from build123d import *

# Parameters (mm, degrees)
CROQUIS1_W               = 30
CROQUIS1_H               = 30
CROQUIS1_W_2             = 26
CROQUIS1_H_2             = 26
SALIENTE_EXTRUIR3_DEPTH  = 230
CROQUIS2_W               = 62.135011277
CROQUIS2_H               = 81.929382736
CORTAR_EXTRUIR3_DEPTH    = 28
CROQUIS3_R               = 2
CORTAR_EXTRUIR9_DEPTH    = 15
CROQUIS4_R               = 2
CORTAR_EXTRUIR10_DEPTH   = 15
CROQUIS5_W               = 30
CROQUIS5_H               = 30
CROQUIS5_W_2             = 26
CROQUIS5_H_2             = 26
SALIENTE_EXTRUIR6_DEPTH  = 12
CROQUIS7_W               = 18.119956634
CROQUIS7_H               = 38.019551867
SALIENTE_EXTRUIR7_DEPTH  = 2
CROQUIS8_W               = 19.256572939
CROQUIS8_H               = 35.130037486
SALIENTE_EXTRUIR8_DEPTH  = 2
CROQUIS9_R               = 2
CORTAR_EXTRUIR11_DEPTH   = 2
CROQUIS10_R              = 2
CORTAR_EXTRUIR12_DEPTH   = 2
CROQUIS11_W              = 68.798737931
CROQUIS11_H              = 42.92716572
CORTAR_EXTRUIR14_DEPTH   = 2
CROQUIS12_R              = 2
SALIENTE_EXTRUIR9_DEPTH  = 2
CROQUIS13_R              = 2
SALIENTE_EXTRUIR10_DEPTH = 2
CROQUIS14_R              = 1.5
CORTAR_EXTRUIR18_DEPTH   = 20
CROQUIS16_W              = 26
CROQUIS16_H              = 26
CROQUIS16_W_2            = 24
CROQUIS16_H_2            = 24
SALIENTE_EXTRUIR11_DEPTH = 212
CROQUIS17_R              = 1.5
CORTAR_EXTRUIR20_DEPTH   = 6
CROQUIS18_R              = 2.5
CORTAR_EXTRUIR21_DEPTH   = 2.25
CROQUIS19_W              = 30
CROQUIS19_H              = 30
CROQUIS19_W_2            = 24
CROQUIS19_H_2            = 24
SALIENTE_EXTRUIR12_DEPTH = 30
CROQUIS20_R              = 2
SALIENTE_EXTRUIR13_DEPTH = 2
CROQUIS21_R              = 2
SALIENTE_EXTRUIR14_DEPTH = 2
CROQUIS22_R              = 2
CORTAR_EXTRUIR22_DEPTH   = 52
CROQUIS23_R              = 2
CORTAR_EXTRUIR23_DEPTH   = 52
CROQUIS24_W              = 34.498036884
CROQUIS24_H              = 39.991384426
CORTAR_EXTRUIR24_DEPTH   = 5


with BuildPart() as part:
    # Croquis1 → Saliente-Extruir3 (new body)
    with BuildSketch(Plane(origin=(0, 0, 0), x_dir=(1, 0, 0), z_dir=(0, 1, 0))):
        Rectangle(CROQUIS1_W, CROQUIS1_H)
        Rectangle(CROQUIS1_W_2, CROQUIS1_H_2, mode=Mode.SUBTRACT)
    extrude(amount=SALIENTE_EXTRUIR3_DEPTH)

    # Croquis2 → Cortar-Extruir3 (cut)
    with BuildSketch(Plane(origin=(0, 230, 0), x_dir=(1, 0, 0), z_dir=(0, 1, 0))):
        with Locations((9.148629236, 2.703749702)):
            Rectangle(CROQUIS2_W, CROQUIS2_H)
    extrude(amount=-CORTAR_EXTRUIR3_DEPTH, mode=Mode.SUBTRACT)

    # Croquis3 → Cortar-Extruir9 (cut)
    with BuildSketch(Plane.XY.offset(15)):
        with Locations((3, 169)):
            Circle(CROQUIS3_R)
        with Locations((-3, 191)):
            Circle(CROQUIS3_R)
        with Locations((-3, 33)):
            Circle(CROQUIS3_R)
        with Locations((3, 11)):
            Circle(CROQUIS3_R)
    extrude(amount=-CORTAR_EXTRUIR9_DEPTH, mode=Mode.SUBTRACT)

    # Croquis4 → Cortar-Extruir10 (cut)
    with BuildSketch(Plane(origin=(0, 0, -15), x_dir=(-1, 0, 0), z_dir=(0, 0, -1))):
        with Locations((-3, 191)):
            Circle(CROQUIS4_R)
        with Locations((3, 169)):
            Circle(CROQUIS4_R)
        with Locations((3, 11)):
            Circle(CROQUIS4_R)
        with Locations((-3, 33)):
            Circle(CROQUIS4_R)
    extrude(amount=-CORTAR_EXTRUIR10_DEPTH, mode=Mode.SUBTRACT)

    # Croquis5 → Saliente-Extruir6 (add)
    with BuildSketch(Plane(origin=(0, 202, 0), x_dir=(1, 0, 0), z_dir=(0, 1, 0))):
        Rectangle(CROQUIS5_W, CROQUIS5_H)
        Rectangle(CROQUIS5_W_2, CROQUIS5_H_2, mode=Mode.SUBTRACT)
    extrude(amount=SALIENTE_EXTRUIR6_DEPTH)

    # Croquis7 → Saliente-Extruir7 (add)
    with BuildSketch(Plane.XY.offset(15)):
        with Locations((-0.954536797, 182.456683749)):
            Rectangle(CROQUIS7_W, CROQUIS7_H)
    extrude(amount=-SALIENTE_EXTRUIR7_DEPTH)

    # Croquis8 → Saliente-Extruir8 (add)
    with BuildSketch(Plane(origin=(0, 0, -15), x_dir=(-1, 0, 0), z_dir=(0, 0, -1))):
        with Locations((1.596533726, 178.910609938)):
            Rectangle(CROQUIS8_W, CROQUIS8_H)
    extrude(amount=-SALIENTE_EXTRUIR8_DEPTH)

    # Croquis9 → Cortar-Extruir11 (cut)
    with BuildSketch(Plane.XY.offset(15)):
        with Locations((-3, 203)):
            Circle(CROQUIS9_R)
        with Locations((3, 181)):
            Circle(CROQUIS9_R)
    extrude(amount=-CORTAR_EXTRUIR11_DEPTH, mode=Mode.SUBTRACT)

    # Croquis10 → Cortar-Extruir12 (cut)
    with BuildSketch(Plane(origin=(0, 0, -15), x_dir=(-1, 0, 0), z_dir=(0, 0, -1))):
        with Locations((-3, 203)):
            Circle(CROQUIS10_R)
        with Locations((3, 181)):
            Circle(CROQUIS10_R)
    extrude(amount=-CORTAR_EXTRUIR12_DEPTH, mode=Mode.SUBTRACT)

    # Croquis11 → Cortar-Extruir14 (cut)
    with BuildSketch(Plane(origin=(0, 214, 0), x_dir=(1, 0, 0), z_dir=(0, 1, 0))):
        with Locations((-6.144488578, -0.254830212)):
            Rectangle(CROQUIS11_W, CROQUIS11_H)
    extrude(amount=-CORTAR_EXTRUIR14_DEPTH, mode=Mode.SUBTRACT)

    # Croquis12 → Saliente-Extruir9 (add)
    with BuildSketch(Plane(origin=(0, 0, -15), x_dir=(-1, 0, 0), z_dir=(0, 0, -1))):
        with Locations((3, 181)):
            Circle(CROQUIS12_R)
        with Locations((-3, 203)):
            Circle(CROQUIS12_R)
    extrude(amount=-SALIENTE_EXTRUIR9_DEPTH)

    # Croquis13 → Saliente-Extruir10 (add)
    with BuildSketch(Plane.XY.offset(15)):
        with Locations((-3, 203)):
            Circle(CROQUIS13_R)
        with Locations((3, 181)):
            Circle(CROQUIS13_R)
    extrude(amount=-SALIENTE_EXTRUIR10_DEPTH)

    # Croquis14 → Cortar-Extruir18 (cut)
    with BuildSketch(Plane.ZY.offset(15)):
        with Locations((0, 204.5)):
            Circle(CROQUIS14_R)
    extrude(amount=-CORTAR_EXTRUIR18_DEPTH, mode=Mode.SUBTRACT)

    # Croquis16 → Saliente-Extruir11 (add)
    with BuildSketch(Plane(origin=(0, 212, 0), x_dir=(1, 0, 0), z_dir=(0, 1, 0))):
        Rectangle(CROQUIS16_W, CROQUIS16_H)
        Rectangle(CROQUIS16_W_2, CROQUIS16_H_2, mode=Mode.SUBTRACT)
    extrude(amount=-SALIENTE_EXTRUIR11_DEPTH)

    # Croquis17 → Cortar-Extruir20 (cut)
    with BuildSketch(Plane.ZY.offset(13)):
        with Locations((0, 204.5)):
            Circle(CROQUIS17_R)
    extrude(amount=-CORTAR_EXTRUIR20_DEPTH, mode=Mode.SUBTRACT)

    # Croquis18 → Cortar-Extruir21 (cut)
    with BuildSketch(Plane.ZY.offset(15)):
        with Locations((0, 204.5)):
            Circle(CROQUIS18_R)
    extrude(amount=-CORTAR_EXTRUIR21_DEPTH, mode=Mode.SUBTRACT)

    # Croquis19 → Saliente-Extruir12 (add)
    with BuildSketch(Plane.XZ):
        Rectangle(CROQUIS19_W, CROQUIS19_H)
        Rectangle(CROQUIS19_W_2, CROQUIS19_H_2, mode=Mode.SUBTRACT)
    extrude(amount=SALIENTE_EXTRUIR12_DEPTH)

    # Croquis20 → Saliente-Extruir13 (add)
    with BuildSketch(Plane.XY.offset(15)):
        with Locations((3, 11)):
            Circle(CROQUIS20_R)
        with Locations((-3, 33)):
            Circle(CROQUIS20_R)
    extrude(amount=-SALIENTE_EXTRUIR13_DEPTH)

    # Croquis21 → Saliente-Extruir14 (add)
    with BuildSketch(Plane(origin=(0, 0, -15), x_dir=(-1, 0, 0), z_dir=(0, 0, -1))):
        with Locations((3, 11)):
            Circle(CROQUIS21_R)
        with Locations((-3, 33)):
            Circle(CROQUIS21_R)
    extrude(amount=-SALIENTE_EXTRUIR14_DEPTH)

    # Croquis22 → Cortar-Extruir22 (cut)
    with BuildSketch(Plane.ZY.offset(15)):
        with Locations((0, -15)):
            Circle(CROQUIS22_R)
    extrude(amount=-CORTAR_EXTRUIR22_DEPTH, mode=Mode.SUBTRACT)

    # Croquis23 → Cortar-Extruir23 (cut)
    with BuildSketch(Plane(origin=(0, 0, -15), x_dir=(-1, 0, 0), z_dir=(0, 0, -1))):
        with Locations((0, -15)):
            Circle(CROQUIS23_R)
    extrude(amount=-CORTAR_EXTRUIR23_DEPTH, mode=Mode.SUBTRACT)

    # Croquis24 → Cortar-Extruir24 (cut)
    with BuildSketch(Plane(origin=(0, -30, 0), x_dir=(-1, 0, 0), z_dir=(0, -1, 0))):
        with Locations((0.940748802, -0.242239461)):
            Rectangle(CROQUIS24_W, CROQUIS24_H)
    extrude(amount=-CORTAR_EXTRUIR24_DEPTH, mode=Mode.SUBTRACT)


solid = part.part
CAD build for the part. Positions are in the model's coordinates, mm. A direction names the side the tool comes from. Give positions to 0.01 mm unless a question says otherwise; leave off trailing zeros. Order: outer loops, then holes, each group sorted by start corner. A loop starts at its lowest first (then second) coordinate and runs counter-clockwise, first axis right, second up. Notation, with made-up numbers: (68.5, 17.5) - (116.5, 17.5) arc R28 cw to (116.5, 46.5) - close; hole circle Ø8 at (22.5, -21.75). An arc over 180 degrees is marked (long way). Answer in a Markdown table with one row per item.
1. Saw through at A-A, the plane z = 8. Give the cut face in (x, y), plus the area to 3 significant figures.
Data:
| item | result |
|---|---|
| outline | (-15, -25) - (-12, -25) - (-12, 212) - (-15, 212) - close; (12, -25) - (15, -25) - (15, 212) - (12, 212) - close |
| area | 1,420 mm² |
2. Pull direction X, two halves, no side cores. Call faces 4 (the flat face through (0, 95, 12)), 5 (the flat face through (15, 95, 0)), 6 (the flat face through (0, 95, 15)), 7 (the flat face through (-12.75, 203, 1)): pulls with the +X half, pulls with the -X half, needs draft (parallel to the pull), parting line crosses it, or undercut.
Data:
| item | result |
|---|---|
| face 4 | undercut |
| face 5 | pulls with the +X half |
| face 6 | needs draft |
| face 7 | pulls with the -X half |
3. Saw through at B-B, the plane y = -15. Give the cut face in (x, z).
Data:
| item | result |
|---|---|
| outline | (-15, -15) - (-2, -15) - (-2, -12) - (-12, -12) - (-12, -2) - (-15, -2) - close; (-15, 2) - (-12, 2) - (-12, 12) - (-2, 12) - (-2, 15) - (-15, 15) - close; (2, -15) - (15, -15) - (15, -2) - (12, -2) - (12, -12) - (2, -12) - close; (2, 12) - (12, 12) - (12, 2) - (15, 2) - (15, 15) - (2, 15) - close |
4. Saw through at D-D, the plane y = 167. Give the cut face in (x, z).
Data:
| item | result |
|---|---|
| outline | (-15, -15) - (15, -15) - (15, 15) - (-15, 15) - close; hole (-12, -12) - (12, -12) - (12, 12) - (-12, 12) - close |
5. Flat gauge pins, fed straight in: pin 1 (4 mm diameter, centred on y = 204.5, z = 0, fed in from -X); pin 2 (3.5 mm diameter, centred on x = 0, y = -15, fed in from +Z). Where does each tip first touch, or does it go through?
Data:
| item | result |
|---|---|
| pin 1 | stops at x = -12.75 |
| pin 2 | passes through |
6. Probe probe 1 along Z at (x, y) = (-8.5, 90); probe 2 along Y at (x, z) = (13.5, 0). List the from-to ranges inside material, lowest first. Write a range as [from, to].
Data:
| item | result |
|---|---|
| probe 1 | z = [-15, -12], [12, 15] |
| probe 2 | y = [-25, -17], [-13, 212] |
7. Tool access for faces 1 (the flat face through (0, 95, -15)), 2 (the cylindrical face through (-14, 207, 0)), 3 (the flat face through (-12, 95, 0)): list every direction of +Z, -Z, +X, -X, +Y, -Y with a clear straight run to the whole face (end or side of a thin tool).
Data:
| item | result |
|---|---|
| face 1 | -Z, +X, -X, +Y, -Y |
| face 2 | -X |
| face 3 | +Y, -Y |
8. Saw through at C-C, the plane x = 9.5. Give the cut face in (y, z).
Data:
| item | result |
|---|---|
| outline | (-25, -15) - (212, -15) - (212, -12) - (-25, -12) - close; (-25, 12) - (212, 12) - (212, 15) - (-25, 15) - close |
